```python
from build123d import *

# Parameters (mm, degrees)
PAD_DEPTH            = 5
SKETCH001_R          = 4.25
POCKET_DEPTH         = 5.001
SKETCH002_R          = 7.5
POCKET001_DEPTH      = 3
SKETCH003_W          = 7.8
SKETCH003_H          = 5
SKETCH003_W_2        = 5
SKETCH003_H_2        = 7.8
PAD001_DEPTH         = 1
FILLET_R             = 0.5
FILLET001_R          = 2
FILLET002_R          = 1
CHAMFER_SIZE         = 0.6
BODY_PLACEMENT_ANGLE = 180


with BuildPart() as part:
    # Sketch → Pad (new body)
    with BuildSketch(Plane.XY):
        Polygon((0, 0), (0, 30), (22, 30), (22, 22), (30, 22), (30, 0), align=None)
    extrude(amount=PAD_DEPTH)

    # Sketch001 (on Face8 of Pad) → Pocket (cut, through all)
    with BuildSketch(Plane.XY.offset(5)):
        with Locations((15, 15)):
            Circle(SKETCH001_R)
    extrude(amount=-POCKET_DEPTH, mode=Mode.SUBTRACT)

    # Sketch002 (on Face5 of Pocket) → Pocket001 (cut)
    with BuildSketch(Plane.XY.offset(5)):
        with Locations((15, 15)):
            Circle(SKETCH002_R)
    extrude(amount=-POCKET001_DEPTH, mode=Mode.SUBTRACT)

    # Sketch003 (on Face4 of Pocket001) → Pad001 (join)
    with BuildSketch(Plane(origin=(0, 0, 0), x_dir=(1, 0, 0), z_dir=(0, 0, -1))):
        with Locations((15, -2.5)):
            Rectangle(SKETCH003_W, SKETCH003_H)
        with Locations((15, -27.5)):
            Rectangle(SKETCH003_W, SKETCH003_H)
        with Locations((2.5, -15)):
            Rectangle(SKETCH003_W_2, SKETCH003_H_2)
        with Locations((27.5, -15)):
            Rectangle(SKETCH003_W_2, SKETCH003_H_2)
    extrude(amount=PAD001_DEPTH)

    # Fillet
    fillet_edges = [part.edges().sort_by_distance(p)[0] for p in [
        (18.9, 0, -0.5),
        (11.1, 0, -0.5),
        (0, 11.1, -0.5),
        (0, 18.9, -0.5),
        (11.1, 30, -0.5),
        (18.9, 30, -0.5),
        (30, 18.9, -0.5),
        (30, 11.1, -0.5),
    ]]
    fillet(fillet_edges, radius=FILLET_R)

    # Fillet001
    fillet001_edges = [part.edges().sort_by_distance(p)[0] for p in [
        (0, 30, 2.5),
        (0, 0, 2.5),
        (30, 0, 2.5),
    ]]
    fillet(fillet001_edges, radius=FILLET001_R)

    # Fillet002
    fillet002_edges = [part.edges().sort_by_distance(p)[0] for p in [
        (22, 30, 2.5),
        (30, 22, 2.5),
    ]]
    fillet(fillet002_edges, radius=FILLET002_R)

    # Chamfer
    chamfer_edges = [part.edges().sort_by_distance(p)[0] for p in [
        (11.5, 30, 5),
        (21.707107, 29.707107, 5),
        (0.585786, 29.414214, 5),
        (22, 25.5, 5),
        (0, 15, 5),
        (25.5, 22, 5),
        (0.585786, 0.585786, 5),
        (29.707107, 21.707107, 5),
        (15, 0, 5),
        (30, 11.5, 5),
        (29.414214, 0.585786, 5),
        (7.5, 15, 5),
    ]]
    chamfer(chamfer_edges, length=CHAMFER_SIZE)


with BuildPart() as part_1:
    # Body placement: moved
    add(part.part.rotate(Axis((0, 0, 0), (0, 1, 0)), BODY_PLACEMENT_ANGLE))


solid = part_1.part
```
Could you check a few things on this model? Use its own coordinates, in mm. A direction names the side the tool comes from. Give positions to 0.01 mm unless a question says otherwise; leave off trailing zeros. Loops run counter-clockwise (first coordinate to the right, second up) from the corner with the lowest first, then second, coordinate; pieces in that order, holes last. Notation, with made-up numbers: (78.25, 62.25) -> (135.25, 62.25) arc R20 cw to (135.25, 86.25) -> close; hole circle Ø6 at (1.25, -20.75). An arc over 180 degrees is marked (long way). Put each result on its own line as item: value.
(1) Thinking about a two-plate mould opening in X: for faces 6 (the face through (-2.7, 11.1, 0.5)), 7 (the face through (-29.165, 0.861, -4.771)), 8 (the face through (-11.88, 11.88, 0)), which applies, pulls with the +X half, pulls with the -X half, needs draft (parallel to the pull), parting line crosses it, or undercut?
Computed:
face 6: needs draft
face 7: pulls with the -X half
face 8: undercut
(2) Please list where these lines run through material, in increasing order: probe 1 along Y at (x, z) = (-15, -0.5); probe 2 along Y at (x, z) = (-17, 0.5); probe 3 along X at (y, z) = (12, 0.25). Write a range as [from, to].
Computed:
probe 1: [0, 10.75], [19.25, 30]
probe 2: [0, 5], [25, 30]
probe 3: [-30, -25], [-5, 0]
(3) For faces 1 (the face through (-27.2, 11.1, 0.5)), 2 (the face through (-25, 22, -2)), 3 (the face through (-18.9, 27.3, 0.5)), 4 (the face through (-18.2, 11.8, -2)), 5 (the face through (-11.1, 27.3, 0.5)), which set-ups out of +Z, -Z, +X, -X, +Y, -Y let a thin tool reach every point of the face, with its end or its side?
Computed:
face 1: +Z, +X, -X, -Y
face 2: +Z, -Z, -X, +Y
face 3: +Z, -X, +Y, -Y
face 4: -Z
face 5: +Z, +X, +Y, -Y
(4) Imagine slicing it at C-C on x = -15. Write out the boundary of the cut face in (y, z), plus the area to 3 significant figures.
Computed:
outline: (0, -4.4) -> (0.6, -5) -> (6.9, -5) -> (7.5, -4.4) -> (7.5, -2) -> (10.75, -2) -> (10.75, 0) -> (5, 0) -> (5, 1) -> (0, 1) -> close; (19.25, -2) -> (22.5, -2) -> (22.5, -4.4) -> (23.1, -5) -> (29.4, -5) -> (30, -4.4) -> (30, 1) -> (25, 1) -> (25, 0) -> (19.25, 0) -> close
area: 97.3 mm^2
(5) I'm going to push flat-ended pins straight in: pin 1 Ø1.1 at (y, z) = (26.5, 0.5) entering from +X; pin 2 Ø7.5 at (x, y) = (-17.5, 16) entering from -Z; pin 3 Ø0.5 at (x, z) = (-28, 0.5) entering from +Y; pin 4 Ø1.5 at (y, z) = (25, -2.5) entering from -X. Where does each tip first touch, or does it pass through?
Computed:
pin 1: x = 0
pin 2: z = -2
pin 3: y = 18.9
pin 4: x = -22
(6) Imagine slicing it at D-D on y = 25.75. Write out the boundary of the cut face in (x, z).
Computed:
outline: (-22, -4.4) -> (-21.4, -5) -> (-0.6, -5) -> (0, -4.4) -> (0, 0) -> (-11.1, 0) -> (-11.1, 1) -> (-18.9, 1) -> (-18.9, 0) -> (-22, 0) -> close
(7) Imagine slicing it at B-B on z = -3. Write out the boundary of the cut face in (x, y).
Computed:
outline: (-30, 2) arc R2 ccw to (-28, 0) -> (-2, 0) arc R2 ccw to (0, 2) -> (0, 28) arc R2 ccw to (-2, 30) -> (-21, 30) arc R1 ccw to (-22, 29) -> (-22, 22) -> (-29, 22) arc R1 ccw to (-30, 21) -> close; hole circle Ø15 at (-15, 15)
(8) Imagine slicing it at A-A on y = 15. Write out the boundary of the cut face in (x, z).
Computed:
outline: (-30, -4.4) -> (-29.4, -5) -> (-23.1, -5) -> (-22.5, -4.4) -> (-22.5, -2) -> (-19.25, -2) -> (-19.25, 0) -> (-25, 0) -> (-25, 1) -> (-30, 1) -> close; (-10.75, -2) -> (-7.5, -2) -> (-7.5, -4.4) -> (-6.9, -5) -> (-0.6, -5) -> (0, -4.4) -> (0, 1) -> (-5, 1) -> (-5, 0) -> (-10.75, 0) -> close
